from build123d import *

# Parameters (mm, degrees)
CHAMFER_1_SIZE      = 0.3
CHAMFER_1_SIZE2     = 0.519615242
FILLET_1_R          = 0.4
FILLET_2_SIZE       = 0.5
FILLET_2_SIZE_2     = 0.8
CUT_EXTRUDE_1_DEPTH = 2


with BuildPart() as part:
    # 草图2 → 旋转1 (revolve)
    with BuildSketch(Plane(origin=(0, 0, 0), x_dir=(0, 0, -1), z_dir=(1, 0, 0)), mode=Mode.PRIVATE) as revolve_1_sk:
        Polygon((-16, 0), (-16, 3.4), (-12, 3.4), (-12, 2), (16, 2), (16, 0), align=None)
    revolve(revolve_1_sk.sketch.rotate(Axis((0, 0, -16), (0, 0, 1)), 90), axis=Axis((0, 0, -16), (0, 0, 1)))

    # 倒角1
    chamfer_1_edges = [part.edges().sort_by_distance(p)[0] for p in [
        (2, 0, -16),
    ]]
    chamfer_1_side = [part.faces().sort_by_distance(p)[0] for p in [
        (2, 0, -2),
    ]]
    chamfer(chamfer_1_edges, length=CHAMFER_1_SIZE, length2=CHAMFER_1_SIZE2, reference=chamfer_1_side[0])

    # 圆角1
    fillet_1_edges = [part.edges().sort_by_distance(p)[0] for p in [
        (3.4, 0, 12),
    ]]
    fillet(fillet_1_edges, radius=FILLET_1_R)

    # 圆角2
    # an asymmetric fillet: 0.8, 0.5 mm, written as the material it takes off along each edge
    with BuildSketch(Plane(origin=(0, 0, 16), x_dir=(-1, 0, 0), z_dir=(0, 1, 0))) as fillet_2_piece_1:
        with BuildLine():
            Bezier((3.4, -FILLET_2_SIZE), (3.4, 0), (3.4 - FILLET_2_SIZE_2, 0), weights=[1, 0.707106781, 1])
            Line((3.4 - FILLET_2_SIZE_2, 0), (3.4, 0))
            Line((3.4, 0), (3.4, -FILLET_2_SIZE))
        make_face()
    revolve(axis=Axis((0, 0, 16), (0, 0, 1)), mode=Mode.SUBTRACT)

    # 草图3 → 切除-拉伸1 (cut)
    with BuildSketch(Plane.XY.offset(16)):
        Polygon((0, 1.732050808), (-1.5, 0.866025404), (-1.5, -0.866025404), (0, -1.732050808), (1.5, -0.866025404), (1.5, 0.866025404), align=None)
    extrude(amount=-CUT_EXTRUDE_1_DEPTH, mode=Mode.SUBTRACT)


solid = part.part
CAD build for the part. Positions are in the model's coordinates, mm. A direction names the side the tool comes from. Round coordinates to 2 decimals unless told otherwise and drop trailing zeros. Write each loop counter-clockwise with the first axis right and the second up, starting at its lowest first coordinate (ties: lowest second). Pieces come first, ordered by that corner, then holes.
(1) Slice it at A-A, the plane z = -1.5. Write the cut outline in (x, y).
(2) Drop flat-ended pins along their axis: P1, Ø4, axis at x = -2.5, z = 4.5, coming from the -Y side; P2, Ø1, axis at x = -0.5, z = -1, coming from the +Y side; P3, Ø0.9, axis at x = 0.5, y = -0.5, coming from the +Z side. Give the stop position or say it passes through.
(3) Probe line 1 along Z through (x, y) = (0.75, -2.25); line 2 along X through (y, z) = (1, -8); line 3 along Z through (x, y) = (-1, -0.75). List the from-to ranges inside material, lowest first.
(4) 3-axis set-ups, long thin cutter, end or side, ignore diameter. For faces 1 (the face through (0, 0, 14)), 2 (the face through (-1, 2, 12)), 3 (the face through (2, 0, 16)): which of +Z, -Z, +X, -X, +Y, -Y reach the whole face in a straight line?
From the geometry:
1. outline: circle Ø4 at (0, 0)
2. P1: stops at y = -1.94
2. P2: stops at y = 2
2. P3: stops at z = 14
3. line 1: z = 12 to 16
3. line 2: x = -1.73 to 1.73
3. line 3: z = -16 to 14
4. face 1: +Z
4. face 2: -Z
4. face 3: +Z, +X, -X, +Y, -Y
